```python
from build123d import *

# Parameters (mm, degrees)
SKETCH1_R                    = 50
BOSS_EXTRUDE1_DEPTH          = 5
F_15_0_15_DIAMETER_HOLE1_D   = 15
F_10_2_10_2_DIAMETER_HOLE1_D = 10.2
M3_CLEARANCE_HOLE1_D         = 3.4
SKETCH9_R                    = 13.5
SKETCH9_R_2                  = 1.5
CUT_EXTRUDE1_DEPTH           = 10
SKETCH10_R                   = 1.65
CUT_EXTRUDE2_DEPTH           = 10
SKETCH13_R                   = 4
CUT_EXTRUDE6_DEPTH           = 10
FILLET1_R                    = 1


with BuildPart() as part:
    # Sketch1 → Boss-Extrude1 (new body)
    with BuildSketch(Plane.XY):
        Circle(SKETCH1_R)
    extrude(amount=BOSS_EXTRUDE1_DEPTH)

    # Ø15.0 (15) Diameter Hole1 (through all)
    with Locations(Plane(origin=(0, 0, 0), x_dir=(-1, 0, 0), z_dir=(0, 0, -1))):
        with Locations((0, 0)):
            Hole(F_15_0_15_DIAMETER_HOLE1_D / 2)

    # Ø10.2 (10.2) Diameter Hole1 (through all)
    with Locations(Plane(origin=(0, 0, 0), x_dir=(-1, 0, 0), z_dir=(0, 0, -1))):
        with Locations((37, 0), (-37, 0), (0, -40)):
            Hole(F_10_2_10_2_DIAMETER_HOLE1_D / 2)

    # M3 Clearance Hole1 (through all)
    with Locations(Plane.XY.offset(5)):
        with Locations((46, 0), (28, 0), (9, -40), (-9, -40), (-46, 0), (-28, 0)):
            Hole(M3_CLEARANCE_HOLE1_D / 2)

    # Sketch9 → Cut-Extrude1 (cut)
    with BuildSketch(Plane.XY.offset(5)):
        with Locations((24.04163056, -24.04163056)):
            Circle(SKETCH9_R)
        with Locations((10.606601718, -10.606601718)):
            Circle(SKETCH9_R_2)
        with Locations((-24.04163056, -24.04163056)):
            Circle(SKETCH9_R)
        with Locations((-10.606601718, -10.606601718)):
            Circle(SKETCH9_R_2)
        with Locations((0, 34)):
            Circle(SKETCH9_R)
        with Locations((0, 15)):
            Circle(SKETCH9_R_2)
    extrude(amount=-CUT_EXTRUDE1_DEPTH, mode=Mode.SUBTRACT)

    # Sketch10 → Cut-Extrude2 (cut)
    with BuildSketch(Plane.XY.offset(5)):
        with Locations((-20.17442319, 27.477446333)):
            Circle(SKETCH10_R)
        with Locations((-29.722400231, 17.23849451)):
            Circle(SKETCH10_R)
        with BuildLine():
            Line((-27.274837591, 48.455628221), (-18.498593172, 40.2716479))
            ThreePointArc((-18.498593172, 40.2716479), (-17.546415771, 38.182285285), (-18.350527147, 36.031591715))
            Line((-18.350527147, 36.031591715), (-38.128479589, 14.822334368))
            ThreePointArc((-38.128479589, 14.822334368), (-40.217842204, 13.870156967), (-42.368535774, 14.674268343))
            Line((-42.368535774, 14.674268343), (-51.144780194, 22.858248664))
            Line((-51.144780194, 22.858248664), (-27.274837591, 48.455628221))
        make_face()
    extrude(amount=-CUT_EXTRUDE2_DEPTH, mode=Mode.SUBTRACT)

    # Sketch13 → Cut-Extrude6 (cut)
    with BuildSketch(Plane.XY.offset(5)):
        with Locations((28.284271247, 28.284271247)):
            Circle(SKETCH13_R)
    extrude(amount=-CUT_EXTRUDE6_DEPTH, mode=Mode.SUBTRACT)

    # Fillet1
    fillet1_edges = [part.edges().sort_by_distance(p)[0] for p in [
        (-22.949421323, 44.422112297, 2.5),
        (-46.456878561, 18.486709669, 2.5),
    ]]
    fillet(fillet1_edges, radius=FILLET1_R)


solid = part.part
```
Input: part model. Units: mm. Frame: model coordinates. A direction names the side the tool comes from. Coordinates: 2 decimals unless noted, no trailing zeros. Write each loop counter-clockwise with the first axis right and the second up, starting at its lowest first coordinate (ties: lowest second). Pieces come first, ordered by that corner, then holes. Notation, with made-up numbers: (42, 88.5) -> (59, 88.5) arc R19 cw to (59, 101.5) -> close; hole circle Ø9 at (19, 8). An arc over 180 degrees is marked (long way). Answer as a JSON object with one key per item and string values.
1. Material intervals for line 1 (Y direction, x = 0, z = 2.75); line 2 (Y direction, x = 6, z = 0.4); line 3 (X direction, y = -23.5, z = 1.25), sorted ascending. Write a range as from..to.
Result set:
{"line 1": "y = -50..-45.1, -34.9..-7.5, 7.5..13.5, 16.5..20.5, 47.5..50", "line 2": "y = -49.64..-4.5, 4.5..21.91, 46.09..49.64", "line 3": "x = -44.13..-37.53, -10.55..10.55, 37.53..44.13"}
2. Section A-A on y = 0. Count the separate pieces of the cut face and the enclosed holes in it, then the cut area to 3 significant figures.
Result set:
{"separate pieces": "8", "enclosed holes": "0", "area": "255 mm2"}
3. First-contact query: P1, Ø2.5, axis at x = -46, y = 0, coming from the -Z side; P2, Ø3, axis at x = 15.5, z = 2.5, coming from the -Y side; P3, Ø3, axis at x = 37, z = 3, coming from the +Y side; P4, Ø2, axis at x = 27, z = 4.5, coming from the +Y side. Flat tips, straight axial feed; report the tip coordinate or a pass-through.
Result set:
{"P1": "passes through", "P2": "stops at y = -48", "P3": "stops at y = 35.21", "P4": "stops at y = 42.71"}
4. Access query for faces 4 (the face through (-43.848, 16.054, 2.535)), 5 (the face through (-44.3, 0.07, 2.47)). Directions: +Z, -Z, +X, -X, +Y, -Y. A direction counts if a zero-diameter tool reaches every point of the face in a straight line with its end or side. Return the directions, or none.
Result set:
{"face 4": "+Z, -Z, +Y", "face 5": "+Z, -Z"}
5. Section D-D on y = -26. Return the cut outline in (x, z).
Result set:
{"outline": "(-42.71, 0) -> (-37.4, 0) -> (-37.4, 5) -> (-42.71, 5) -> close; (-10.68, 0) -> (10.68, 0) -> (10.68, 5) -> (-10.68, 5) -> close; (37.4, 0) -> (42.71, 0) -> (42.71, 5) -> (37.4, 5) -> close"}
6. Section C-C on x = -25. Return the cut outline in (y, z), then the cut area to 3 significant figures.
Result set:
{"outline": "(-43.3, 0) -> (-37.51, 0) -> (-37.51, 5) -> (-43.3, 5) -> close; (-10.58, 0) -> (28.9, 0) -> (28.9, 5) -> (-10.58, 5) -> close", "area": "226 mm2"}
7. Mould query, pull axis Y, two halves, no side actions, for faces 1 (the face through (-40.18, 13.87, 2.54)), 2 (the face through (10, 1, 0)), 3 (the face through (-28.101, 25.575, 2.535)). Classes: released by +Y, released by -Y, zero draft, split by the parting line, or undercut.
Result set:
{"face 1": "released by +Y", "face 2": "zero draft", "face 3": "undercut"}
